from build123d import *

# Parameters (mm, degrees)
F1_DEPTH  = 10
F2_R      = 7
F2_R_2    = 3
F3_DEPTH  = 1
F4_DEPTH  = 6
F5_SIZE   = 0.5
F6_W      = 2.1
F6_H      = 20
F8_DEPTH  = 8
F7_W      = 2.1
F7_H      = 20
F9_DEPTH  = 8
F10_R     = 2.25
F11_DEPTH = 28.101
F10_W     = 3
F10_H     = 2.7
F12_DEPTH = 1.5


with BuildPart() as f1:
    # F0 (on Top) → F1 (new body, symmetric)
    with BuildSketch(Plane.XY):
        Polygon((-20.5, -18.5), (20.5, -18.5), (20.5, 16.4531469345), (18.5, 18.5), (-14, 18.5), (-17.5, 15.5), (-20.5, 15.5), align=None)
    extrude(amount=F1_DEPTH, both=True)

    # F2 (on face) → F3 (join)
    with BuildSketch(Plane(origin=(0, 18.5, 0), x_dir=(-1, 0, 0), z_dir=(0, 1, 0))):
        with Locations((-10, 0)):
            Circle(F2_R)
        with Locations((-10, 0)):
            Circle(F2_R_2, mode=Mode.SUBTRACT)
    extrude(amount=F3_DEPTH)

    # F4 (add): a face of the model
    f4_faces = [f1.faces().sort_by_distance(p)[0] for p in [
        (10, 18.5, 0),
    ]]
    extrude(f4_faces, amount=F4_DEPTH)

    # F5
    f5_edges = [f1.edges().sort_by_distance(p)[0] for p in [
        (17, 19.5, 0),
    ]]
    chamfer(f5_edges, length=F5_SIZE)

    # F6 (on face) → F8 (join)
    with BuildSketch(Plane(origin=(-20.5, 0, 0), x_dir=(0, -1, 0), z_dir=(-1, 0, 0))):
        with Locations((-8.55, 0)):
            Rectangle(F6_W, F6_H)
    extrude(amount=F8_DEPTH)

    # F7 (on face) → F9 (join)
    with BuildSketch(Plane.YZ.offset(20.5)):
        with Locations((8.55, 0)):
            Rectangle(F7_W, F7_H)
    extrude(amount=F9_DEPTH)

    # F10 (on face) → F11 (cut, through all)
    with BuildSketch(Plane(origin=(0, 9.6, 0), x_dir=(-1, 0, 0), z_dir=(0, 1, 0))):
        with Locations((-25.25, 5.75)):
            Circle(F10_R)
        with Locations((-25.25, -5.75)):
            Circle(F10_R)
        with Locations((25.25, -5.75)):
            Circle(F10_R)
        with Locations((25.25, 5.75)):
            Circle(F10_R)
    extrude(amount=-F11_DEPTH, mode=Mode.SUBTRACT)

    # F10 (on face) → F12 (join)
    with BuildSketch(Plane(origin=(0, 9.6, 0), x_dir=(-1, 0, 0), z_dir=(0, 1, 0))):
        with Locations((-22, 0)):
            Rectangle(F10_W, F10_H)
        with Locations((22, 0)):
            Rectangle(F10_W, F10_H)
    extrude(amount=F12_DEPTH)


solid = f1.part
Input: part model. Units: mm. Frame: model coordinates. A direction names the side the tool comes from. Coordinates: 2 decimals unless noted, no trailing zeros. Loops run counter-clockwise (first coordinate to the right, second up) from the corner with the lowest first, then second, coordinate; pieces in that order, holes last. Notation, with made-up numbers: (-32.5, -37.75) -> (10.5, -37.75) arc R34 ccw to (10.5, -6.75) -> close; hole circle Ø1 at (-3.75, 40). An arc over 180 degrees is marked (long way). Write item = value, one per line. Start each with the question number.
Item 1: Cut plane B-B, the plane z = -9. Return loops of the section in (x, y), plus the area to 3 significant figures.
Item 2: Cut plane C-C, the plane x = 10. Return loops of the section in (y, z), plus the area to 3 significant figures.
Item 3: First-contact query: P1, Ø4, axis at x = -25.25, z = 5.75, coming from the +Y side; P2, Ø6, axis at y = -7.5, z = -3, coming from the +X side; P3, Ø10, axis at y = 19.5, z = -5, coming from the -X side; P4, Ø4.5, axis at y = 12.5, z = -2, coming from the -X side. Flat tips, straight axial feed; report the tip coordinate or a pass-through.
Item 4: Material intervals for line 1 (Z direction, x = 25.25, y = 8.65); line 2 (X direction, y = 3.5, z = -2.5); line 3 (Y direction, x = -22, z = 6.5), sorted ascending.
Item 5: Mould query, pull axis X, two halves, no side actions, for faces 1 (the face through (23.104, 8.565, 6.426)), 2 (the face through (0, 0, 10)), 3 (the face through (23.5, 10, 0)). Classes: pulls with the +X half, pulls with the -X half, needs draft (parallel to the pull), parting line crosses it, or undercut.
Item 6: Reachability of faces 4 (the face through (24, 7.5, 0)), 5 (the face through (7, 19.5, -1)), 6 (the face through (-23.5, 10, 0)), 7 (the face through (-24, 7.5, 0)) from +Z, -Z, +X, -X, +Y, -Y: full face, straight path, thin tool, end or side. Return the list, or none.
Item 7: Cut plane A-A, the plane x = -25.25. Return loops of the section in (y, z).
Item 8: Cut plane D-D, the plane y = 14. Return loops of the section in (x, z).
Ans:
q1.outline = (-28.5, 7.5) -> (-20.5, 7.5) -> (-20.5, -18.5) -> (20.5, -18.5) -> (20.5, 7.5) -> (28.5, 7.5) -> (28.5, 9.6) -> (20.5, 9.6) -> (20.5, 16.45) -> (18.5, 18.5) -> (-14, 18.5) -> (-17.5, 15.5) -> (-20.5, 15.5) -> (-20.5, 9.6) -> (-28.5, 9.6) -> close
q1.area = 1,530 mm²
q2.outline = (-18.5, -10) -> (18.5, -10) -> (18.5, -7) -> (19, -7) -> (19.5, -6.5) -> (19.5, -3) -> (24.5, -3) -> (24.5, 3) -> (19.5, 3) -> (19.5, 6.5) -> (19, 7) -> (18.5, 7) -> (18.5, 10) -> (-18.5, 10) -> close
q2.area = 784 mm²
q3.P1 = through
q3.P2 = 20.5
q3.P3 = -20.5
q3.P4 = -23.5
q4.line_1 = -10 to -8, -3.5 to 3.5, 8 to 10
q4.line_2 = -20.5 to 20.5
q4.line_3 = 7.5 to 9.6
q5.face_1 = undercut
q5.face_2 = needs draft
q5.face_3 = pulls with the +X half
q6.face_4 = +Z, -Z, +X, -Y
q6.face_5 = +Y
q6.face_6 = +Z, -Z, -X, +Y
q6.face_7 = +Z, -Z, -X, -Y
q7.outline = (7.5, -10) -> (9.6, -10) -> (9.6, -8) -> (7.5, -8) -> close; (7.5, -3.5) -> (9.6, -3.5) -> (9.6, 3.5) -> (7.5, 3.5) -> close; (7.5, 8) -> (9.6, 8) -> (9.6, 10) -> (7.5, 10) -> close
q8.outline = (-20.5, -10) -> (20.5, -10) -> (20.5, 10) -> (-20.5, 10) -> close
